Verification items for the finished model (mm, model axes). Coordinates: 2 decimals unless noted, no trailing zeros. Order: outer loops, then holes, each group sorted by start corner. A loop starts at its lowest first (then second) coordinate and runs counter-clockwise, first axis right, second up. Notation, with made-up numbers: M 32,-21 L 55,-21 A26 cw 55,-4 Z; hole C 51,43.5 d9. An arc over 180 degrees is marked long. Return JSON: item names as keys, results as strings. Group by question number.
1. Material ranges on line 1 along X through (y, z) = (43.5, 14); line 2 along Z through (x, y) = (1.5, 34.5); line 3 along Z through (x, y) = (-0.5, 52), recorded low to high.
2. Section check D-D, the plane x = 4. Record the cut outline in (y, z), plus the area to 3 significant figures.
3. Section check C-C, the plane x = 0.75. Record the cut outline in (y, z).
4. Gauge pin test, flat end, axial feed: pin 1 (1.5 mm diameter, centred on x = 5, y = 12, fed in from +Z). Record the tip position at first contact, or that the pin passes through.
5. Section check B-B, the plane y = 29.5. Record the cut outline in (x, z).
6. Section check A-A, the plane z = -14. Record the cut outline in (x, y), plus the area to 3 significant figures.
7. Mould release check, pull along X, two halves, no side actions. Record for faces 1 (the cylindrical face through (-0.54, 28.1, 16.44)), 2 (the flat face through (7, 28, -4)), 3 (the flat face through (0, 28, -21)), 4 (the flat face through (-7, 28, 0)): +X half, -X half, draft (parallel to the pull), parting line (faces both ways), or undercut.
```python
from build123d import *

# Parameters (mm, degrees)
SKETCH_1_R      = 2.5
EXTRUDE_1_DEPTH = 57


with BuildPart() as part:
    # 草图1 → 凸台-拉伸1 (new body)
    with BuildSketch(Plane(origin=(0, 0, 0), x_dir=(1, 0, 0), z_dir=(0, 1, 0))):
        with BuildLine():
            Line((-7, 21), (7, 21))
            Line((7, 21), (7, -14))
            ThreePointArc((7, -14), (4.949747468, -18.949747468), (0, -21))
            Line((0, -21), (-7, -21))
            Line((-7, -21), (-7, 21))
        make_face()
        with Locations((0, 14)):
            Circle(SKETCH_1_R, mode=Mode.SUBTRACT)
        with Locations((0, -14)):
            Circle(SKETCH_1_R, mode=Mode.SUBTRACT)
    extrude(amount=EXTRUDE_1_DEPTH)


solid = part.part
```
Answers follow:
{
 "1": {"line 1": "-7 to -2.5, 2.5 to 7", "line 2": "-21 to -16, -12 to 12, 16 to 20.84", "line 3": "-21 to -16.45, -11.55 to 11.55, 16.45 to 21"},
 "2": {"outline": "M 0,-21 L 57,-21 L 57,19.74 L 0,19.74 Z", "area": "2,320 mm^2"},
 "3": {"outline": "M 0,-21 L 57,-21 L 57,-16.38 L 0,-16.38 Z; M 0,-11.62 L 57,-11.62 L 57,11.62 L 0,11.62 Z; M 0,16.38 L 57,16.38 L 57,20.96 L 0,20.96 Z"},
 "4": {"pin 1": "z = 19.56"},
 "5": {"outline": "M -7,-21 L 7,-21 L 7,14 A7 ccw 0,21 L -7,21 Z; hole C 0,-14 d5; hole C 0,14 d5"},
 "6": {"outline": "M -7,0 L -2.5,0 L -2.5,57 L -7,57 Z; M 2.5,0 L 7,0 L 7,57 L 2.5,57 Z", "area": "513 mm^2"},
 "7": {"face 1": "undercut", "face 2": "+X half", "face 3": "draft", "face 4": "-X half"}
}
